For this review, take the finished solid that the model builds, in its own axes (mm). Face numbers are marked on the shaded views. A direction names the side the tool comes from. Coordinates: 2 decimals unless noted, no trailing zeros. Loops run counter-clockwise (first coordinate to the right, second up) from the corner with the lowest first, then second, coordinate; pieces in that order, holes last.
```python
from build123d import *

# Parameters (mm, degrees)
F2_W        = 75
F2_H        = 100
F3_DEPTH    = 50
F4_T        = -2
F5_W        = 20
F5_H        = 2
F6_DEPTH    = 4
F7_T1_DEPTH = 26.4948974279


# Not quite as in the source:
# - a fillet or chamfer that OpenCascade refuses, or shapes differently, is made with other operations: its cross-section is extruded or revolved along the edge and cut away or added


with BuildPart() as f3:
    # F2 (on Top) → F3 (new body)
    with BuildSketch(Plane.XY):
        Rectangle(F2_W, F2_H)
    extrude(amount=-F3_DEPTH)

    # F4
    f4_openings = [f3.faces().sort_by_distance(p)[0] for p in [
        (0, 0, 0),
    ]]
    offset(amount=F4_T, openings=f4_openings)

    # F5 (on face) → F6 (join)
    with BuildSketch(Plane.XZ.offset(50)):
        with Locations((0, -49)):
            Rectangle(F5_W, F5_H)
    extrude(amount=F6_DEPTH)

    # F7: fillet of radius 5 on 2 edges, made by hand

    # F7_s2 → F7_t1 (cut)
    with BuildSketch(Plane.XY.offset(-62.2474487139)):
        with BuildLine():
            ThreePointArc((10, -50), (8.2632981746, -52.8729833462), (5.1010205144, -54))
            Line((5.1010205144, -54), (10, -54))
            Line((10, -54), (10, -50))
        make_face()
        with BuildLine():
            ThreePointArc((-10, -50), (-8.2632981746, -52.8729833462), (-5.1010205144, -54))
            Line((-5.1010205144, -54), (-10, -54))
            Line((-10, -54), (-10, -50))
        make_face()
    extrude(amount=F7_T1_DEPTH, mode=Mode.SUBTRACT)


solid = f3.part
```
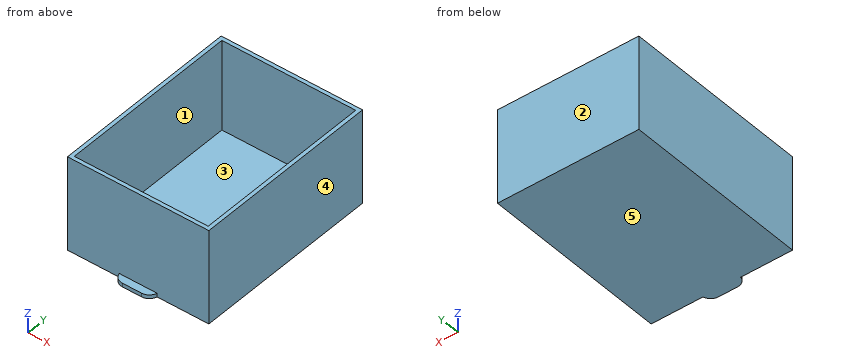
Q1. Machinability: for the marked faces 1 and 2, which of the approach directions +Z, -Z, +X, -X, +Y, -Y give a long, thin tool a straight path to every point of the face, cutting with its end or side? Answer none if there is none.
Q2. Wall thickness on probe 1 along X at (y, z) = (-42.5, -19); probe 2 along Y at (x, z) = (9.5, -20); probe 3 along Z at (x, y) = (-25.5, -29.5): over which ranges is each line inside the solid? List them lowest first.
Q3. Consider section A-A (z = -20). State the section outline as (x, y) points.
Q4. Consider section C-C (y = 12). State the section outline as (x, z) points, then the cut area to 3 significant figures.
Q5. The part is to be moulded in two halves that separate along X. For the marked faces 3, 4 and 5, say which applies: +X half, -X half, draft (parallel to the pull), parting line (faces both ways), or undercut.
Q6. Consider section B-B (x = -2). State the section outline as (y, z) points, then the cut area to 3 significant figures.
Q7. For pin 1 Ø4 at (x, z) = (18.5, -34) entering from -Y; pin 2 Ø21.5 at (x, y) = (-16, 19.5) entering from +Z, all flat-tipped, find the tip position at first contact; note any pin that passes through.
Q8. Consider section D-D (x = 17.5). State the section outline as (y, z) points.
Model answer:
1. face 1: +Z
1. face 2: +Z, -Z, +X, -X, +Y
2. probe 1: x = -37.5 to -35.5, 35.5 to 37.5
2. probe 2: y = -50 to -48, 48 to 50
2. probe 3: z = -50 to -48
3. outline: (-37.5, -50) - (37.5, -50) - (37.5, 50) - (-37.5, 50) - close; hole (-35.5, -48) - (35.5, -48) - (35.5, 48) - (-35.5, 48) - close
4. outline: (-37.5, -50) - (37.5, -50) - (37.5, 0) - (35.5, 0) - (35.5, -48) - (-35.5, -48) - (-35.5, 0) - (-37.5, 0) - close
4. area: 342 mm2
5. face 3: undercut
5. face 4: +X half
5. face 5: draft
6. outline: (-54, -50) - (50, -50) - (50, 0) - (48, 0) - (48, -48) - (-48, -48) - (-48, 0) - (-50, 0) - (-50, -48) - (-54, -48) - close
6. area: 400 mm2
7. pin 1: stops at y = -50
7. pin 2: stops at z = -48
8. outline: (-50, -50) - (50, -50) - (50, 0) - (48, 0) - (48, -48) - (-48, -48) - (-48, 0) - (-50, 0) - close
